Study the drawing (mm; zero at the part's minimum x, y, z) and answer. A direction names the side the tool comes from. Give positions to 0.01 mm unless a question says otherwise; leave off trailing zeros. Order: outer loops, then holes, each group sorted by start corner. A loop starts at its lowest first (then second) coordinate and runs counter-clockwise, first axis right, second up.
Item 1: Given pin 1 Ø1.6 at (x, z) = (0.5, 12) entering from -Y; pin 2 Ø1 at (x, z) = (41, 61) entering from -Y; pin 3 Ø8 at (x, y) = (38, 59) entering from +Z, each flat-ended and moving along its own axis, determine where each tip first touches the part or whether it passes through.
Item 2: A cutting plane is placed at C-C (y = 62). Write down the section's boundary in (x, z).
Item 3: Find the intervals of material crossed by line 1 along Y through (x, z) = (46.5, 150.5); line 2 along Z through (x, y) = (65.5, 21.5), in increasing order.
Item 4: A cutting plane is placed at D-D (z = 86). Write down the section's boundary in (x, y).
Item 5: A cutting plane is placed at B-B (x = 23). Write down the section's boundary in (y, z).
Item 6: A cutting plane is placed at A-A (z = 146.5). Write down the section's boundary in (x, y).
Item 7: The mould has two halves that part along X. Classify the marked faces 1, 2, 3 and 4: +X half, -X half, draft (parallel to the pull), parting line (faces both ways), or undercut.
Item 8: Which of the six approach directions +Z, -Z, +X, -X, +Y, -Y give full straight-line access (tool end or side, diameter ignored) to the marked faces 5 and 6?
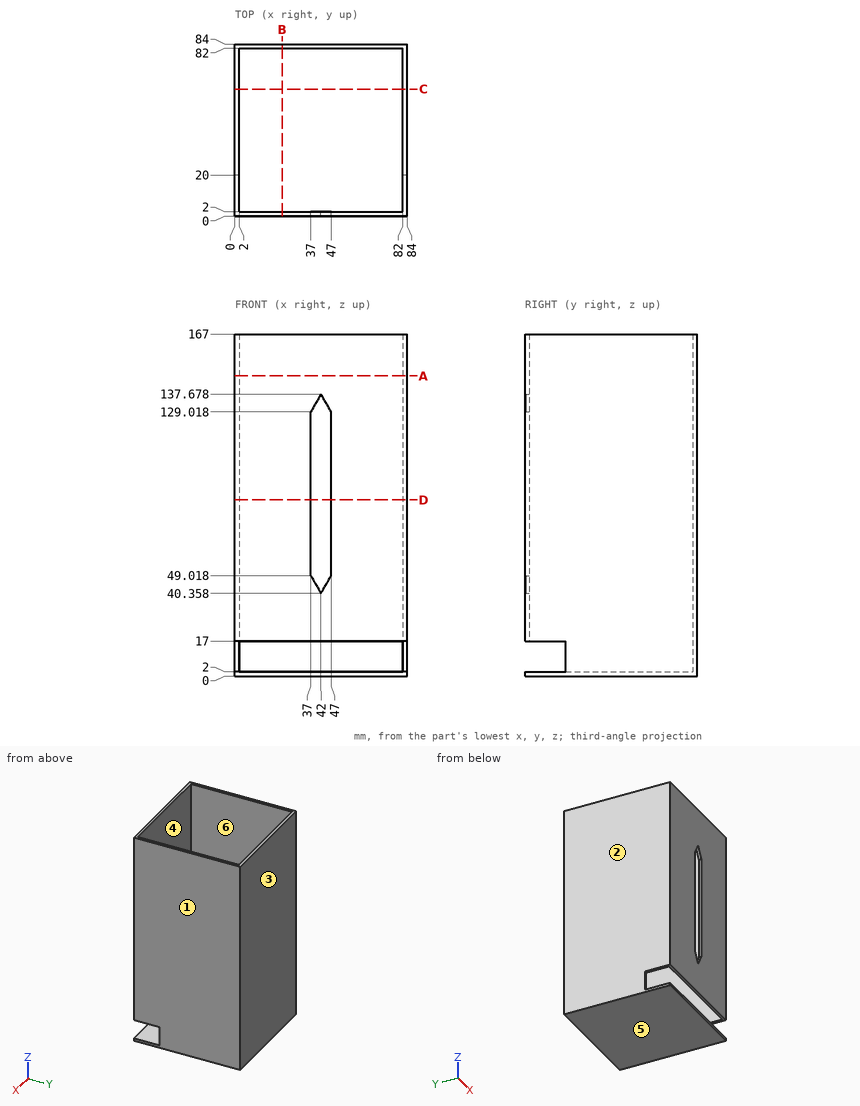
Response values:
1. pin 1: stops at y = 20
1. pin 2: stops at y = 82
1. pin 3: stops at z = 2
2. outline: (0, 0) - (84, 0) - (84, 167) - (82, 167) - (82, 2) - (2, 2) - (2, 167) - (0, 167) - close
3. line 1: y = 0 to 2, 82 to 84
3. line 2: z = 0 to 2
4. outline: (0, 0) - (37, 0) - (37, 2) - (2, 2) - (2, 82) - (82, 82) - (82, 2) - (47, 2) - (47, 0) - (84, 0) - (84, 84) - (0, 84) - close
5. outline: (0, 0) - (84, 0) - (84, 167) - (82, 167) - (82, 2) - (0, 2) - close; (0, 17) - (2, 17) - (2, 167) - (0, 167) - close
6. outline: (0, 0) - (84, 0) - (84, 84) - (0, 84) - close; hole (2, 2) - (82, 2) - (82, 82) - (2, 82) - close
7. face 1: +X half
7. face 2: -X half
7. face 3: draft
7. face 4: undercut
8. face 5: -Z, +X, -X, +Y, -Y
8. face 6: +Z
